```python
from build123d import *

# Parameters (mm, degrees)
SKETCH_1_W          = 30.8
SKETCH_1_H          = 54
EXTRUDE_1_DEPTH     = 5
SKETCH_2_W          = 30.8
SKETCH_2_H          = 4
EXTRUDE_2_DEPTH     = 8
SKETCH_3_R          = 1.5
CUT_EXTRUDE_1_DEPTH = 5
SKETCH_4_W          = 30.8
SKETCH_4_H          = 3
EXTRUDE_3_DEPTH     = 8
SKETCH_5_W          = 30.8
SKETCH_5_H          = 1.45
EXTRUDE_4_DEPTH     = 1
SKETCH_6_W          = 30.8
SKETCH_6_H          = 1.45
EXTRUDE_5_DEPTH     = 1
SKETCH_7_W          = 5
SKETCH_7_H          = 22
EXTRUDE_6_DEPTH     = 8


with BuildPart() as part:
    # 草图1 → 凸台-拉伸1 (new body)
    with BuildSketch(Plane.XY):
        Rectangle(SKETCH_1_W, SKETCH_1_H)
    extrude(amount=EXTRUDE_1_DEPTH)

    # 草图2 → 凸台-拉伸2 (add)
    with BuildSketch(Plane(origin=(0, 0, 0), x_dir=(-1, 0, 0), z_dir=(0, 0, -1))):
        with Locations((0, -25)):
            Rectangle(SKETCH_2_W, SKETCH_2_H)
    extrude(amount=EXTRUDE_2_DEPTH)

    # 草图3 → 切除-拉伸1 (cut, through all)
    with BuildSketch(Plane(origin=(0, -23, 0), x_dir=(1, 0, 0), z_dir=(0, 1, 0))):
        with Locations((10.4, 4)):
            Circle(SKETCH_3_R)
        with Locations((-10.4, 4)):
            Circle(SKETCH_3_R)
    extrude(amount=-CUT_EXTRUDE_1_DEPTH, mode=Mode.SUBTRACT)

    # 草图4 → 凸台-拉伸3 (add)
    with BuildSketch(Plane(origin=(0, 0, 0), x_dir=(-1, 0, 0), z_dir=(0, 0, -1))):
        with Locations((0, 25.5)):
            Rectangle(SKETCH_4_W, SKETCH_4_H)
        with Locations((0, 5.5)):
            Rectangle(SKETCH_4_W, SKETCH_4_H)
    extrude(amount=EXTRUDE_3_DEPTH)

    # 草图5 → 凸台-拉伸4 (add)
    with BuildSketch(Plane(origin=(0, 7, 0), x_dir=(1, 0, 0), z_dir=(0, 1, 0))):
        with Locations((0, 7.275)):
            Rectangle(SKETCH_5_W, SKETCH_5_H)
    extrude(amount=EXTRUDE_4_DEPTH)

    # 草图6 → 凸台-拉伸5 (add)
    with BuildSketch(Plane.XZ.offset(-24)):
        with Locations((0, -7.275)):
            Rectangle(SKETCH_6_W, SKETCH_6_H)
    extrude(amount=EXTRUDE_5_DEPTH)

    # 草图7 → 凸台-拉伸6 (add)
    with BuildSketch(Plane(origin=(0, 0, 0), x_dir=(-1, 0, 0), z_dir=(0, 0, -1))):
        with Locations((0, -7)):
            Rectangle(SKETCH_7_W, SKETCH_7_H)
    extrude(amount=EXTRUDE_6_DEPTH)


solid = part.part
```
Can you work these out from the model? Positions are in its coordinate system, mm. A direction names the side the tool comes from. Round coordinates to 2 decimals unless told otherwise and drop trailing zeros. Loops run counter-clockwise (first coordinate to the right, second up) from the corner with the lowest first, then second, coordinate; pieces in that order, holes last. Notation, with made-up numbers: (88.5, 18) -> (144.5, 18) arc R19 cw to (144.5, 43) -> close; hole circle Ø7 at (6, 53). An arc over 180 degrees is marked (long way). One line per item, written item: value. Start each with the question number.
1. If we section it at B-B, the plane z = -1: Write out the boundary of the cut face in (x, y), then the cut area to 3 significant figures.
2. If we mould it in two halves opening along Z, with no side actions, what happens to faces 1 (the flat face through (-0.2, 7.5, -6.55)), 2 (the flat face through (0, -25, -8)), 3 (the flat face through (0, 24, -3)), 4 (the flat face through (0, 23, -7))? For each: pulls with the +Z half, pulls with the -Z half, needs draft (parallel to the pull), parting line crosses it, or undercut.
3. If we section it at C-C, the plane z = -4: Write out the boundary of the cut face in (x, y), then the cut area to 3 significant figures.
4. For faces 5 (the flat face through (-9, 4, -4)), 6 (the cylindrical face through (-8.97, -24.97, -4.45)), 7 (the flat face through (0, -18, -4)), 8 (the flat face through (0, -27, -1)), 9 (the flat face through (2.5, -7, -4)), which set-ups out of +Z, -Z, +X, -X, +Y, -Y let a thin tool reach every point of the face, with its end or its side?
5. If we section it at A-A, the plane x = 10.4: Write out the boundary of the cut face in (y, z), then the cut area to 3 significant figures.
6. If I drill on probe 1 along Y at (x, z) = (7, -1); probe 2 along X at (y, z) = (-25.95, -4); probe 3 along Y at (x, z) = (-2, -5.5), over which ranges is the centre line in solid material (lowest first)?
7. For pin 1 (4 mm diameter, centred on y = 20.5, z = -5.5, fed in from +X); pin 2 (2.5 mm diameter, centred on y = -3, z = -4.5, fed in from -X); pin 3 (1.8 mm diameter, centred on x = -10.4, z = -4, fed in from -Y); pin 4 (2.5 mm diameter, centred on y = -4, z = -5.5, fed in from +X), each with a flat end and sliding along its axis, tell me the tip position at first contact or that it passes through.
8. If we section it at D-D, the plane x = 5.5: Write out the boundary of the cut face in (y, z).
Calculated:
1. outline: (-15.4, -27) -> (15.4, -27) -> (15.4, -23) -> (-15.4, -23) -> close; (-15.4, 4) -> (-2.5, 4) -> (-2.5, -18) -> (2.5, -18) -> (2.5, 4) -> (15.4, 4) -> (15.4, 7) -> (-15.4, 7) -> close; (-15.4, 24) -> (15.4, 24) -> (15.4, 27) -> (-15.4, 27) -> close
1. area: 418 mm²
2. face 1: undercut
2. face 2: pulls with the -Z half
2. face 3: undercut
2. face 4: needs draft
3. outline: (-15.4, -27) -> (-11.9, -27) -> (-11.9, -23) -> (-15.4, -23) -> close; (-15.4, 4) -> (-2.5, 4) -> (-2.5, -18) -> (2.5, -18) -> (2.5, 4) -> (15.4, 4) -> (15.4, 7) -> (-15.4, 7) -> close; (-15.4, 24) -> (15.4, 24) -> (15.4, 27) -> (-15.4, 27) -> close; (-8.9, -27) -> (8.9, -27) -> (8.9, -23) -> (-8.9, -23) -> close; (11.9, -27) -> (15.4, -27) -> (15.4, -23) -> (11.9, -23) -> close
3. area: 394 mm²
4. face 5: -Z, -X
4. face 6: -Y
4. face 7: -Z, +X, -X
4. face 8: +Z, -Z, +X, -X, -Y
4. face 9: -Z, +X
5. outline: (-27, -8) -> (-23, -8) -> (-23, -5.5) -> (-27, -5.5) -> close; (-27, -2.5) -> (-23, -2.5) -> (-23, 0) -> (4, 0) -> (4, -8) -> (8, -8) -> (8, -6.55) -> (7, -6.55) -> (7, 0) -> (24, 0) -> (24, -6.55) -> (23, -6.55) -> (23, -8) -> (27, -8) -> (27, 5) -> (-27, 5) -> close
5. area: 341 mm²
6. probe 1: y = -27 to -23, 4 to 7, 24 to 27
6. probe 2: x = -15.4 to -11.9, -8.9 to 8.9, 11.9 to 15.4
6. probe 3: y = -27 to -23, -18 to 7, 24 to 27
7. pin 1: passes through
7. pin 2: stops at x = -2.5
7. pin 3: stops at y = 4
7. pin 4: stops at x = 2.5
8. outline: (-27, -8) -> (-23, -8) -> (-23, 0) -> (4, 0) -> (4, -8) -> (8, -8) -> (8, -6.55) -> (7, -6.55) -> (7, 0) -> (24, 0) -> (24, -6.55) -> (23, -6.55) -> (23, -8) -> (27, -8) -> (27, 5) -> (-27, 5) -> close
